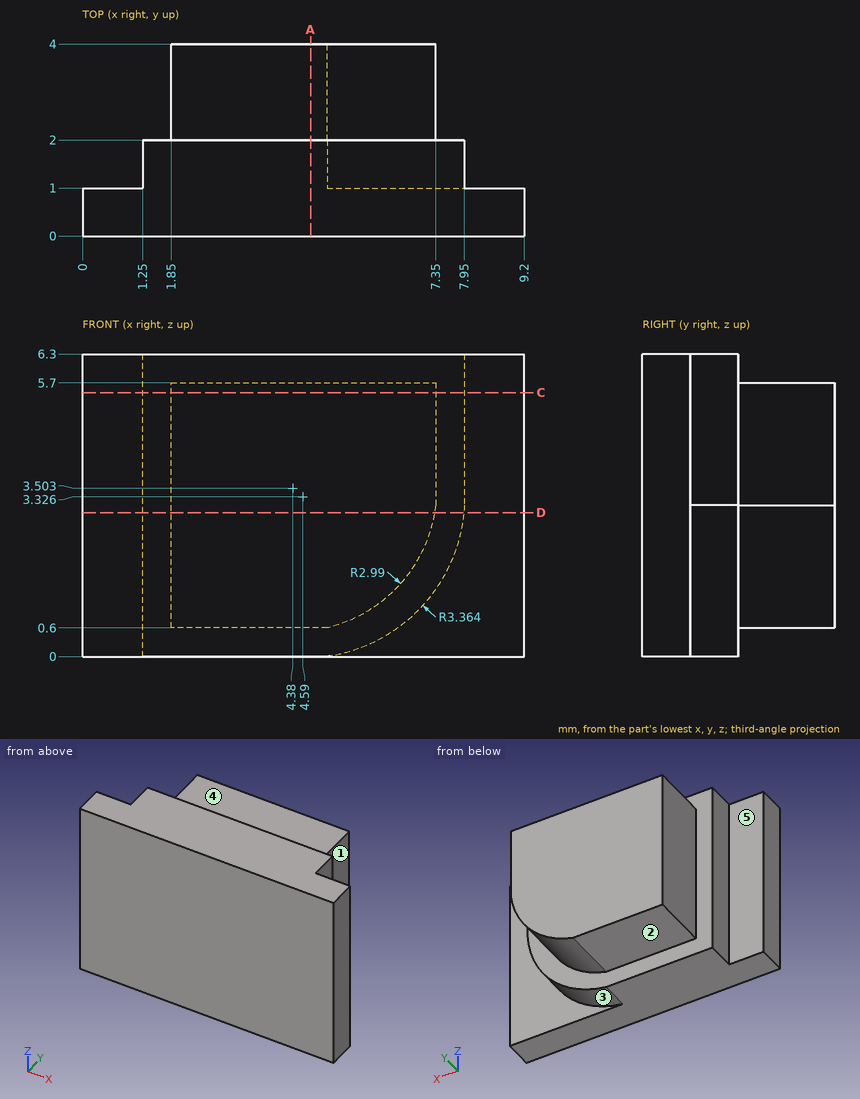
The drawing under review shows one solid part. Ordinate dimensions are in mm from its lowest x, y, z. A direction names the side the tool comes from. Coordinates: 2 decimals unless noted, no trailing zeros. Write each loop counter-clockwise with the first axis right and the second up, starting at its lowest first coordinate (ties: lowest second). Pieces come first, ordered by that corner, then holes. Notation, with made-up numbers: M 56,3.25 L 84,3.25 A35 ccw 84,41.25 Z; hole C 24,-2.5 d1. An arc over 180 degrees is marked long. Put each result on its own line as item: value.
1) Clearance check with flat-ended pins moving along their axes: pin 1 Ø0.8 at (y, z) = (1.5, 5) entering from +X; pin 2 Ø1 at (x, z) = (1, 3.5) entering from +Y; pin 3 Ø0.6 at (x, y) = (3.5, 2.5) entering from +Z. State where each tip first meets the part, or that it passes through.
Computed:
pin 1: stops at x = 7.95
pin 2: stops at y = 2
pin 3: stops at z = 5.7
2) Add section C-C on z = 5.5. Give the boundary of the cut face in (x, y).
Computed:
outline: M 0,0 L 9.2,0 L 9.2,1 L 7.95,1 L 7.95,2 L 7.35,2 L 7.35,4 L 1.85,4 L 1.85,2 L 1.25,2 L 1.25,1 L 0,1 Z
3) Wall thickness on probe 1 along X at (y, z) = (1.9, 5.5); probe 2 along X at (y, z) = (3.2, 5); probe 3 along Z at (x, y) = (3.5, 2.4): over which ranges is each line inside the solid? List them lowest first. Write a range as [from, to].
Computed:
probe 1: x = [1.25, 7.95]
probe 2: x = [1.85, 7.35]
probe 3: z = [0.6, 5.7]
4) For the marked faces 1, 2, 3, 4 and 5, list the 3-axis set-ups (+Z, -Z, +X, -X, +Y, -Y) from which the entire face can be reached by the end or side of a thin tool; tool diameter is ignored.
Computed:
face 1: +Z, -Z, +X, +Y
face 2: -Z, +X, -X, +Y
face 3: -Z, +X, +Y
face 4: +Z, +X, -X, +Y
face 5: +Z, -Z, -X, +Y
5) Add section D-D on z = 3. Give the boundary of the cut face in (x, y).
Computed:
outline: M 0,0 L 9.2,0 L 9.2,1 L 7.94,1 L 7.94,2 L 7.33,2 L 7.33,4 L 1.85,4 L 1.85,2 L 1.25,2 L 1.25,1 L 0,1 Z
6) Add section A-A on x = 4.75. Give the boundary of the cut face in (y, z).
Computed:
outline: M 0,0 L 2,0 L 2,0.6 L 4,0.6 L 4,5.7 L 2,5.7 L 2,6.3 L 0,6.3 Z
